```python
from build123d import *

# Parameters (mm, degrees)
F0_R     = 19.4994564254
F1_DEPTH = 31.75
F2_R     = 5.08
F3_R     = 14.3450562753
F4_DEPTH = 38.354
F6_R     = 13.3830864671
F7_DEPTH = 2.032
F8_R     = 12.9352143756
F9_DEPTH = 2.286


# Not quite as in the source:
# - a fillet or chamfer that OpenCascade refuses, or shapes differently, is made with other operations: its cross-section is extruded or revolved along the edge and cut away or added


with BuildPart() as f1:
    # F0 (on Top) → F1 (new body)
    with BuildSketch(Plane.XY):
        Circle(F0_R)
    extrude(amount=F1_DEPTH)

    # F2
    f2_edges = [f1.edges().sort_by_distance(p)[0] for p in [
        (-19.499456, 0, 31.75),
    ]]
    fillet(f2_edges, radius=F2_R)

    # F3 (on Top) → F4 (join)
    with BuildSketch(Plane.XY):
        Circle(F3_R)
    extrude(amount=F4_DEPTH)

    # F5: fillet of radius 10.4245741623 on 1 edges, made by hand

    # F5_s1 → F5_t2 (revolve, cut)
    with BuildSketch(Plane.XZ):
        with BuildLine():
            ThreePointArc((14.3450562753, 31.75), (10.5128533097, 36.5462583521), (4.6458315879, 38.354))
            Line((4.6458315879, 38.354), (14.3450562753, 38.354))
            Line((14.3450562753, 38.354), (14.3450562753, 31.75))
        make_face()
    revolve(axis=Axis((0, 0, 38.354), (0, 0, 1)), mode=Mode.SUBTRACT)

    # F6 (on Right) → F7 (join)
    with BuildSketch(Plane.YZ):
        with Locations((0, 51.0602071881)):
            Circle(F6_R)
    extrude(amount=F7_DEPTH)

    # F8 (on Right) → F9 (join)
    with BuildSketch(Plane.YZ):
        with Locations((0, 51.4653660357)):
            Circle(F8_R)
    extrude(amount=-F9_DEPTH)


solid = f1.part
```
Input: part model. Units: mm. Frame: model coordinates. A direction names the side the tool comes from. Give positions to 0.01 mm unless a question says otherwise; leave off trailing zeros. Write each loop counter-clockwise with the first axis right and the second up, starting at its lowest first coordinate (ties: lowest second). Pieces come first, ordered by that corner, then holes. Notation, with made-up numbers: (76, 85.5) - (90, 85.5) arc R22 ccw to (90, 115.5) - close; hole circle Ø7 at (17, 2). An arc over 180 degrees is marked (long way). Write item = value, one per line. Start each with the question number.
1. Access query for faces 1 (the flat face through (0, -4, 39)), 2 (the cylindrical face through (18.6, 5.86, 13.15)), 3 (the flat face through (3, 0, 38.354)). Directions: +Z, -Z, +X, -X, +Y, -Y. A direction counts if a zero-diameter tool reaches every point of the face in a straight line with its end or side. Return the directions, or none.
2. Section query A-A, the plane z = 5. Output: boundary loops of the cut face in (x, y).
3. Section query B-B, the plane z = 54. Output: boundary loops of the cut face in (x, y).
4. First-contact query: pin 1 Ø10 at (x, z) = (-0.5, 49) entering from +Y; pin 2 Ø3 at (x, y) = (-9.5, 11.5) entering from -Z; pin 3 Ø1.5 at (y, z) = (-11, 7) entering from -X; pin 4 Ø1 at (y, z) = (-8.5, 23.5) entering from -X. Flat tips, straight axial feed; report the tip coordinate or a pass-through.
5. Mould query, pull axis Z, two halves, no side actions, for faces 4 (the flat face through (-2.286, 0, 52)), 5 (the flat face through (0, 0, 0)), 6 (the flat face through (-2, 0, 38.354)). Classes: released by +Z, released by -Z, zero draft, split by the parting line, or undercut.
6. Ray query, L1, parallel to X at y = 1, z = 42; L2, parallel to Z at x = 3, y = 3; L3, parallel to Z at x = 14.5, y = -1. Return the intervals inside material, ascending.
Check sheet entries:
q1.face_1 = -X
q1.face_2 = +Z, -Z
q1.face_3 = +Z, +X, +Y, -Y
q2.outline = circle Ø39 at (0, 0)
q3.outline = (-2.29, -12.68) - (0, -12.68) - (0, -13.06) - (2.03, -13.06) - (2.03, 13.06) - (0, 13.06) - (0, 12.68) - (-2.29, 12.68) - close
q4.pin_1 = 13.38
q4.pin_2 = 0
q4.pin_3 = -16.59
q4.pin_4 = -17.78
q5.face_4 = zero draft
q5.face_5 = released by -Z
q5.face_6 = undercut
q6.L1 = -2.29 to 2.03
q6.L2 = 0 to 38.35
q6.L3 = 0 to 31.75
